```python
from build123d import *

# Parameters (mm, degrees)
SKETCH1_W                        = 66.494000054
SKETCH1_H                        = 30.426
BOSS_EXTRUDE1_DEPTH              = 5.842
F_11_64_0_17188_DIAMETER_HOLE1_D = 4.365752
F_0_257_DIAMETER_HOLE1_D         = 6.5278
BOSS_EXTRUDE3_DEPTH              = 5.842
F_0_257_DIAMETER_HOLE3_D         = 6.5278
SKETCH13_W                       = 8.999982
SKETCH13_H                       = 6.35
CUT_EXTRUDE1_DEPTH               = 105.431017222
CHAMFER1_SIZE                    = 2.54
BOSS_EXTRUDE6_DEPTH              = 5.842
FILLET1_R                        = 3.175
FILLET2_R                        = 1.5875
FILLET3_R                        = 1.5875
BOSS_EXTRUDE7_DEPTH              = 5.842
FILLET4_R                        = 3.175
FILLET5_R                        = 6.35
FILLET6_R                        = 3.175
CUT_EXTRUDE3_DEPTH               = 116.434993398
CUT_EXTRUDE4_DEPTH               = 116.434993398
FILLET10_R                       = 3.175
SKETCH29_W                       = 87.204685613
SKETCH29_H                       = 5.08
CUT_EXTRUDE6_DEPTH               = 116.434993398
FILLET12_R                       = 6.35


with BuildPart() as part:
    # Sketch1 → Boss-Extrude1 (new body)
    with BuildSketch(Plane.XY):
        with BuildLine():
            Line((-75.493982054, 0), (-75.493982054, 30.426))
            ThreePointArc((-75.493982054, 30.426), (-74.175965205, 33.607974151), (-70.993991054, 34.925991))
            Line((-70.993991054, 34.925991), (4.499991, 34.925991))
            ThreePointArc((4.499991, 34.925991), (7.681965151, 33.607974151), (8.999982, 30.426))
            Line((8.999982, 30.426), (8.999982, 0))
            Line((8.999982, 0), (11.100760908, -11.565106481))
            ThreePointArc((11.100760908, -11.565106481), (7.160083484, -18.61606843), (-0.513638035, -16.094362457))
            Line((-0.513638035, -16.094362457), (-7.847000027, -4.499991))
            Line((-7.847000027, -4.499991), (-58.647000027, -4.499991))
            Line((-58.647000027, -4.499991), (-65.980362019, -16.094362457))
            ThreePointArc((-65.980362019, -16.094362457), (-73.654083538, -18.61606843), (-77.594760962, -11.565106481))
            Line((-77.594760962, -11.565106481), (-75.493982054, 0))
        make_face()
        with Locations((-33.247000027, 15.213)):
            Rectangle(SKETCH1_W, SKETCH1_H, mode=Mode.SUBTRACT)
    extrude(amount=BOSS_EXTRUDE1_DEPTH)

    # 11/64 (0.17188) Diameter Hole1 (through all)
    with Locations(Plane.XY.offset(5.842)):
        with Locations((-70.993991054, 24.357), (-70.993991054, 6.069)):
            f_11_64_0_17188_diameter_hole1 = Hole(F_11_64_0_17188_DIAMETER_HOLE1_D / 2)

    # Mirror1: 11/64 (0.17188) Diameter Hole1 across plane
    add(f_11_64_0_17188_diameter_hole1.mirror(Plane.ZY.offset(33.247000027)), mode=Mode.SUBTRACT)

    # F (0.257) Diameter Hole1 (through all)
    with Locations(Plane.XY.offset(5.842)):
        with Locations((-71.347000027, -12.7)):
            f_0_257_diameter_hole1 = Hole(F_0_257_DIAMETER_HOLE1_D / 2)

    # Mirror2: F (0.257) Diameter Hole1 across plane
    add(f_0_257_diameter_hole1.mirror(Plane.ZY.offset(33.247000027)), mode=Mode.SUBTRACT)

    # Sketch10 → Boss-Extrude3 (add)
    with BuildSketch(Plane.XY.offset(5.842)):
        with BuildLine():
            Line((-95.26734363, 20.592874824), (-73.384544712, 34.314048933))
            Line((-73.384544712, 34.314048933), (-68.603437396, 34.314048933))
            Line((-68.603437396, 34.314048933), (-75.493982054, 30.426))
            Line((-75.493982054, 30.426), (-75.493982054, 22.368465679))
            Line((-75.493982054, 22.368465679), (-85.597223399, 16.03342901))
            ThreePointArc((-85.597223399, 16.03342901), (-85.544000054, 15.213), (-85.597223399, 14.39257099))
            Line((-85.597223399, 14.39257099), (-75.493982054, 8.057534321))
            Line((-75.493982054, 8.057534321), (-75.493982054, 0))
            Line((-75.493982054, 0), (-75.901345831, -2.242599371))
            Line((-75.901345831, -2.242599371), (-95.26734363, 9.833125176))
            ThreePointArc((-95.26734363, 9.833125176), (-98.244000054, 15.213), (-95.26734363, 20.592874824))
        make_face()
    extrude(amount=-BOSS_EXTRUDE3_DEPTH)

    # F (0.257) Diameter Hole3 (through all)
    with Locations(Plane.XY.offset(5.842)):
        with Locations((-91.894000054, 15.213)):
            Hole(F_0_257_DIAMETER_HOLE3_D / 2)

    # Sketch13 → Cut-Extrude1 (cut, through all)
    with BuildSketch(Plane.XY.offset(5.842)):
        with Locations((4.499991, 15.213)):
            Rectangle(SKETCH13_W, SKETCH13_H)
    extrude(amount=-CUT_EXTRUDE1_DEPTH, mode=Mode.SUBTRACT)

    # Chamfer1
    chamfer1_edges = [part.edges().sort_by_distance(p)[0] for p in [
        (0, 12.038, 2.921),
        (0, 18.388, 2.921),
    ]]
    chamfer(chamfer1_edges, length=CHAMFER1_SIZE)

    # Sketch22 → Boss-Extrude6 (add)
    with BuildSketch(Plane.XY.offset(5.842)):
        Polygon((8.999982, 18.388), (8.999982, 24.738), (21.699982, 21.563), (21.699982, 8.863), (8.999982, 5.688), (8.999982, 12.038), (15.349982, 12.038), (15.349982, 18.388), align=None)
    extrude(amount=-BOSS_EXTRUDE6_DEPTH)

    # Fillet1
    fillet1_edges = [part.edges().sort_by_distance(p)[0] for p in [
        (8.999982, 24.738, 2.921),
        (21.699982, 21.563, 2.921),
        (21.699982, 8.863, 2.921),
        (8.999982, 5.688, 2.921),
    ]]
    fillet(fillet1_edges, radius=FILLET1_R)

    # Fillet2
    fillet2_edges = [part.edges().sort_by_distance(p)[0] for p in [
        (15.349982, 18.388, 2.921),
        (15.349982, 12.038, 2.921),
    ]]
    fillet(fillet2_edges, radius=FILLET2_R)

    # Fillet3
    # the kernel refuses this fillet: 1.5875 mm, written as the material it adds along each edge
    with BuildSketch(Plane(origin=(-75.493982054, 8.057534321, 5.842), x_dir=(0, 1, 0), z_dir=(0, 0, -1))) as fillet3_piece_1:
        with BuildLine():
            CenterArc((FILLET3_R * 1.80735498388, -FILLET3_R), FILLET3_R, 90, 122.088950954)
            Line((FILLET3_R * 0.960130602163, -FILLET3_R * 1.53123520876), (0, 0))
            Line((0, 0), (FILLET3_R * 1.80735498388, 0))
        make_face()
    extrude(amount=5.842)
    with BuildSketch(Plane(origin=(-75.493982054, 22.368465679, 5.842), x_dir=(0, -1, 0), z_dir=(0, 0, -1))) as fillet3_piece_2:
        with BuildLine():
            CenterArc((FILLET3_R * 1.80735498388, FILLET3_R), FILLET3_R, 147.911049046, 122.088950954)
            Line((FILLET3_R * 0.960130602163, FILLET3_R * 1.53123520876), (0, 0))
            Line((0, 0), (FILLET3_R * 1.80735498388, 0))
        make_face()
    extrude(amount=5.842)
    with BuildSketch(Plane(origin=(-85.597223399, 14.39257099, 5.842), x_dir=(0.06319147380474219, 0.9980014216615047, 0), z_dir=(0, 0, -1))) as fillet3_piece_3:
        with BuildLine():
            CenterArc((0.946995123, 1.584009043), FILLET3_R, 208.465932253, 57.73363863)
            Line((-0.448577196, 0.827349177), (0, 0))
            ThreePointArc((0, 0), (0.420886721, 0.013963828), (0.841773443, 0))
        make_face()
    extrude(amount=5.842)
    with BuildSketch(Plane(origin=(-85.597223399, 16.03342901, 5.842), x_dir=(0.8472243817163825, 0.5312352087590706, 0), z_dir=(0, 0, -1))) as fillet3_piece_4:
        with BuildLine():
            CenterArc((0.94113132, 1.5875), FILLET3_R, 212.26636137, 57.73363863)
            ThreePointArc((-0.401219641, 0.7400036), (-0.18833421, 0.376657465), (0, 0))
            Line((0, 0), (0.94113132, 0))
        make_face()
    extrude(amount=5.842)

    # Sketch24 → Boss-Extrude7 (add)
    with BuildSketch(Plane(origin=(0, 0, 0), x_dir=(-1, 0, 0), z_dir=(0, 0, -1))):
        Polygon((57.037580054, 48.794391), (57.037580054, 41.275991), (62.879580054, 41.275991), (62.879580054, 34.925991), (70.993991054, 34.925991), (73.259602339, 34.314048933), (73.384544712, 34.314048933), (75.493982054, 32.991368176), (69.229580054, 60.325991), (62.879580054, 60.325991), (62.879580054, 53.975991), (57.037580054, 53.975991), align=None)
        Polygon((0.200579946, 60.325991), (-6.149420054, 60.325991), (-21.699982, 19.08403491), (-9.699273994, 22.99974755), (0.200579946, 34.925991), (0.200579946, 41.275991), (6.042579946, 41.275991), (6.042579946, 48.794391), (6.042579946, 53.975991), (0.200579946, 53.975991), align=None)
    boss_extrude7 = extrude(amount=-BOSS_EXTRUDE7_DEPTH)

    # Fillet4
    fillet4_edges = [part.edges().sort_by_distance(p)[0] for p in [
        (-75.493982054, 32.991368176, 2.921),
        (-69.229580054, 60.325991, 2.921),
    ]]
    fillet(fillet4_edges, radius=FILLET4_R)

    # Fillet5
    fillet5_edges = [part.edges().sort_by_distance(p)[0] for p in [
        (20.909565621, 21.180313983, 2.921),
    ]]
    fillet(fillet5_edges, radius=FILLET5_R)

    # Fillet6
    fillet6_edges = [part.edges().sort_by_distance(p)[0] for p in [
        (6.149420054, 60.325991, 2.921),
    ]]
    fillet(fillet6_edges, radius=FILLET6_R)

    # Sketch26 → Cut-Extrude3 (cut, through all)
    with BuildSketch(Plane(origin=(0, 0, 0), x_dir=(-1, 0, 0), z_dir=(0, 0, -1))):
        Polygon((89.149059257, -30.603913947), (-16.445159676, -30.603913947), (-16.445159676, -4.499991), (-16.445159676, 1.604517455), (-8.999982, 1.604517455), (-8.999982, -4.499991), (75.901345831, -4.499991), (75.901345831, -2.242599371), (89.149059257, -2.242599371), (89.149059257, -4.499991), align=None)
    extrude(amount=-CUT_EXTRUDE3_DEPTH, mode=Mode.SUBTRACT)

    # Mirror3: Boss-Extrude7 across plane
    add(boss_extrude7.mirror(Plane(origin=(0, 15.213, 0), x_dir=(0, 0, 1), z_dir=(0, -1, 0))))

    # Sketch28 → Cut-Extrude4 (cut, through all)
    with BuildSketch(Plane(origin=(0, 0, 0), x_dir=(-1, 0, 0), z_dir=(0, 0, -1))):
        Polygon((75.050615589, -4.499991), (75.901345831, -2.242599371), (75.901345831, -4.499991), align=None)
    extrude(amount=-CUT_EXTRUDE4_DEPTH, mode=Mode.SUBTRACT)

    # Fillet10
    fillet10_edges = [part.edges().sort_by_distance(p)[0] for p in [
        (6.149420054, -29.899991, 2.921),
        (-75.050615589, -4.499991, 2.921),
        (-69.229580054, -29.899991, 2.921),
        (-75.901345831, -2.242599371, 2.921),
    ]]
    fillet(fillet10_edges, radius=FILLET10_R)

    # Sketch29 → Cut-Extrude6 (cut, through all)
    with BuildSketch(Plane.XY.offset(5.842)):
        with Locations((-32.135383003, -27.359991)):
            Rectangle(SKETCH29_W, SKETCH29_H)
    extrude(amount=-CUT_EXTRUDE6_DEPTH, mode=Mode.SUBTRACT)

    # Fillet12
    fillet12_edges = [part.edges().sort_by_distance(p)[0] for p in [
        (8.064868839, -24.819991, 2.921),
        (-70.393787161, -24.819991, 2.921),
    ]]
    fillet(fillet12_edges, radius=FILLET12_R)


solid = part.part
```
Check sheet for the modelled part. Datum: model origin and axes. Units: mm. A direction names the side the tool comes from. Round coordinates to 2 decimals unless told otherwise and drop trailing zeros. Loops run counter-clockwise (first coordinate to the right, second up) from the corner with the lowest first, then second, coordinate; pieces in that order, holes last. Notation, with made-up numbers: (-4, -36) - (16, -36) arc R22 cw to (16, -21) - close; hole circle Ø2 at (54.25, 32). An arc over 180 degrees is marked (long way). Answer as a JSON object with one key per item and string values. Group by question number.
Q1. Sectioned sample at A-A, the plane x = -29. Enter the section's corners in (y, z), plus the area to 3 significant figures.
Q2. Scan lines: line 1 along Y through (x, z) = (-6, 0.4); line 2 along Y through (x, z) = (-7.5, 1.65); line 3 along Y through (x, z) = (6.5, 0.8). Record each from-to range of solid material in increasing order. Write a range as [from, to].
Q3. Sectioned sample at D-D, the plane z = 4. Count the separate pieces of the cut face and the enclosed holes in it, plus the area to 3 significant figures.
Q4. Sectioned sample at B-B, the plane x = -59. Enter the section's corners in (y, z).
Q5. Mould release check, pull along Y, two halves, no side actions. Record for faces 1 (the face through (15.35, 15, 3)), 2 (the face through (-69.244, -23.473, 2.88)), 3 (the face through (-65, 60.326, 3)): released by +Y, released by -Y, zero draft, split by the parting line, or undercut.
Q6. Sectioned sample at C-C, the plane y = -6.5. Enter the section's corners in (x, z).
Q7. Gauge pin test, flat ends, axial feed: P1, Ø3, axis at x = -3, z = 2, coming from the -Y side; P2, Ø3, axis at x = -45, z = 2, coming from the -Y side; P3, Ø3, axis at y = 37.5, z = 3.5, coming from the -X side. Record the tip position at first contact, or that the pin passes through.
Q8. Set-up check for faces 4 (the face through (-57.038, -17, 3)), 5 (the face through (-57.038, 48, 3)), 6 (the face through (-62.88, -8, 3)), 7 (the face through (7.33, -23.66, 2.96)), 8 (the face through (-98.243, 15.123, 2.962)): record each of +Z, -Z, +X, -X, +Y, -Y from which the full face is reachable in a straight line by a thin tool's end or side.
Solution:
{
 "1": {"outline": "(-4.5, 0) - (0, 0) - (0, 5.84) - (-4.5, 5.84) - close; (30.43, 0) - (34.93, 0) - (34.93, 5.84) - (30.43, 5.84) - close", "area": "52.6 mm²"},
 "2": {"line 1": "y = [-23.55, -10.85], [-4.5, 0], [30.43, 34.93], [41.28, 53.98]", "line 2": "y = [-4.5, 0], [30.43, 34.93]", "line 3": "y = [-24.16, 5.19], [6.94, 12.04], [18.39, 23.48], [25.23, 59.05]"},
 "3": {"separate pieces": "1", "enclosed holes": "7", "area": "3,170 mm²"},
 "4": {"outline": "(-23.55, 0) - (-10.85, 0) - (-10.85, 5.84) - (-23.55, 5.84) - close; (-4.5, 0) - (0, 0) - (0, 5.84) - (-4.5, 5.84) - close; (30.43, 0) - (34.93, 0) - (34.93, 5.84) - (30.43, 5.84) - close; (41.28, 0) - (53.98, 0) - (53.98, 5.84) - (41.28, 5.84) - close"},
 "5": {"face 1": "undercut", "face 2": "released by -Y", "face 3": "released by +Y"},
 "6": {"outline": "(-74.59, 0) - (-62.88, 0) - (-62.88, 5.84) - (-74.59, 5.84) - close; (-0.2, 0) - (14.97, 0) - (14.97, 5.84) - (-0.2, 5.84) - close"},
 "7": {"P1": "stops at y = -23.55", "P2": "stops at y = -4.5", "P3": "stops at x = -74.8"},
 "8": {"face 4": "+Z, -Z, -Y", "face 5": "+Z, -Z, +Y", "face 6": "+Z, -Z", "face 7": "+Z, -Z, +X, -Y", "face 8": "+Z, -Z, -X"}
}
